Here's how the part is built. I have some questions about the finished solid (model axes, mm). A direction names the side the tool comes from. Give positions to 0.01 mm unless a question says otherwise; leave off trailing zeros. Order: outer loops, then holes, each group sorted by start corner. A loop starts at its lowest first (then second) coordinate and runs counter-clockwise, first axis right, second up. Notation, with made-up numbers: (88, 37) - (110, 37) arc R9 cw to (110, 43) - close; hole circle Ø4 at (11, 40). An arc over 180 degrees is marked (long way). One line per question, with ' | ' between items.
from build123d import *

# Parameters (mm, degrees)
SKETCH1_W                                 = 16
SKETCH1_H                                 = 16
BASE_DEPTH                                = 55
SKETCH2_W                                 = 2
SKETCH2_H                                 = 16
RODSLOT_DEPTH                             = 17
F_5_1_5_1_FREE_HOLE_FOR_SCREW_D           = 5.1
F_5_1_5_1_FREE_HOLE_FOR_SCREW_DEPTH       = 7.5
F_5_1_5_1_FREE_HOLE_FOR_SCREW_CSINK_D     = 6.1
F_5_1_5_1_FREE_HOLE_FOR_SCREW_CSINK_ANGLE = 90
F_5_1_5_1_FREE_HOLE_FOR_SCREW_TIP         = 1.056244584
M5X0_8_TAPPED_HOLE_FOR_ROD_SCREW_D        = 4.2
M5X0_8_TAPPED_HOLE_FOR_ROD_SCREW_DEPTH    = 7.6381927
M5X0_8_TAPPED_HOLE_FOR_ROD_SCREW_TIP      = 1.2618073
F_10_2_10_2_ROD_HOLE_D                    = 10.2
SKETCH13_W                                = 20
SKETCH13_H                                = 2
ROD2SLOT_DEPTH                            = 17
F_10_2_10_2_ROD2_HOLE_D                   = 10.2
F_5_1_5_1_DIAMETER_HOLE1_D                = 5.1
F_5_1_5_1_DIAMETER_HOLE1_DEPTH            = 7.5
F_5_1_5_1_DIAMETER_HOLE1_CSINK_D          = 6.1
F_5_1_5_1_DIAMETER_HOLE1_CSINK_ANGLE      = 90
F_5_1_5_1_DIAMETER_HOLE1_TIP              = 1.056244584
M5X0_8_TAPPED_HOLE1_D                     = 4.2
M5X0_8_TAPPED_HOLE1_DEPTH                 = 7.6381927
M5X0_8_TAPPED_HOLE1_TIP                   = 1.2618073


with BuildPart() as part:
    # Sketch1 → Base (new body)
    with BuildSketch(Plane.XY):
        Rectangle(SKETCH1_W, SKETCH1_H)
    extrude(amount=BASE_DEPTH)

    # Sketch2 → RodSlot (cut, through all)
    with BuildSketch(Plane(origin=(0, 8, 0), x_dir=(1, 0, 0), z_dir=(0, 1, 0))):
        with Locations((0, -47)):
            Rectangle(SKETCH2_W, SKETCH2_H)
    extrude(amount=-RODSLOT_DEPTH, mode=Mode.SUBTRACT)

    # Ø5.1 (5.1) free hole for screw
    with Locations(Plane(origin=(8, 0, 0), x_dir=(0, 0, -1), z_dir=(1, 0, 0))):
        with Locations((-50, 0)):
            CounterSinkHole(F_5_1_5_1_FREE_HOLE_FOR_SCREW_D / 2, F_5_1_5_1_FREE_HOLE_FOR_SCREW_CSINK_D / 2, depth=F_5_1_5_1_FREE_HOLE_FOR_SCREW_DEPTH, counter_sink_angle=F_5_1_5_1_FREE_HOLE_FOR_SCREW_CSINK_ANGLE)
            with Locations((0, 0, -(F_5_1_5_1_FREE_HOLE_FOR_SCREW_DEPTH + F_5_1_5_1_FREE_HOLE_FOR_SCREW_TIP / 2))):  # 135° drill point
                Cone(0, F_5_1_5_1_FREE_HOLE_FOR_SCREW_D / 2, F_5_1_5_1_FREE_HOLE_FOR_SCREW_TIP, mode=Mode.SUBTRACT)

    # M5x0.8 Tapped Hole for rod screw
    with Locations(Plane.ZY.offset(8)):
        with Locations((50, 0)):
            Hole(M5X0_8_TAPPED_HOLE_FOR_ROD_SCREW_D / 2, depth=M5X0_8_TAPPED_HOLE_FOR_ROD_SCREW_DEPTH)
            with Locations((0, 0, -(M5X0_8_TAPPED_HOLE_FOR_ROD_SCREW_DEPTH + M5X0_8_TAPPED_HOLE_FOR_ROD_SCREW_TIP / 2))):  # 118° drill point
                Cone(0, M5X0_8_TAPPED_HOLE_FOR_ROD_SCREW_D / 2, M5X0_8_TAPPED_HOLE_FOR_ROD_SCREW_TIP, mode=Mode.SUBTRACT)

    # Ø10.2 (10.2) Rod Hole (through all)
    with Locations(Plane(origin=(0, 8, 0), x_dir=(1, 0, 0), z_dir=(0, 1, 0))):
        with Locations((0, -35)):
            Hole(F_10_2_10_2_ROD_HOLE_D / 2)

    # Sketch13 → Rod2Slot (cut, through all)
    with BuildSketch(Plane.ZY.offset(8)):
        with Locations((10, 0)):
            Rectangle(SKETCH13_W, SKETCH13_H)
    extrude(amount=-ROD2SLOT_DEPTH, mode=Mode.SUBTRACT)

    # Ø10.2 (10.2) Rod2 Hole (through all)
    with Locations(Plane(origin=(-8, 0, 0), x_dir=(0, 1, 0), z_dir=(-1, 0, 0))):
        with Locations((0, -20)):
            Hole(F_10_2_10_2_ROD2_HOLE_D / 2)

    # Ø5.1 (5.1) Diameter Hole1
    with Locations(Plane(origin=(0, 8, 0), x_dir=(0, 0, -1), z_dir=(0, 1, 0))):
        with Locations((-5, 0)):
            CounterSinkHole(F_5_1_5_1_DIAMETER_HOLE1_D / 2, F_5_1_5_1_DIAMETER_HOLE1_CSINK_D / 2, depth=F_5_1_5_1_DIAMETER_HOLE1_DEPTH, counter_sink_angle=F_5_1_5_1_DIAMETER_HOLE1_CSINK_ANGLE)
            with Locations((0, 0, -(F_5_1_5_1_DIAMETER_HOLE1_DEPTH + F_5_1_5_1_DIAMETER_HOLE1_TIP / 2))):  # 135° drill point
                Cone(0, F_5_1_5_1_DIAMETER_HOLE1_D / 2, F_5_1_5_1_DIAMETER_HOLE1_TIP, mode=Mode.SUBTRACT)

    # M5x0.8 Tapped Hole1
    with Locations(Plane(origin=(0, -8, 0), x_dir=(-1, 0, 0), z_dir=(0, -1, 0))):
        with Locations((0, -5)):
            Hole(M5X0_8_TAPPED_HOLE1_D / 2, depth=M5X0_8_TAPPED_HOLE1_DEPTH)
            with Locations((0, 0, -(M5X0_8_TAPPED_HOLE1_DEPTH + M5X0_8_TAPPED_HOLE1_TIP / 2))):  # 118° drill point
                Cone(0, M5X0_8_TAPPED_HOLE1_D / 2, M5X0_8_TAPPED_HOLE1_TIP, mode=Mode.SUBTRACT)


solid = part.part
1) I want a section at D-D (z = 50). List the corners of the cut face in (x, y) for me.
Model answer:
outline: (-8, -8) - (-1, -8) - (-1, -2.1) - (-8, -2.1) - close; (-8, 2.1) - (-1, 2.1) - (-1, 8) - (-8, 8) - close; (1, -8) - (8, -8) - (8, -3.05) - (7.5, -2.55) - (1, -2.55) - close; (1, 2.55) - (7.5, 2.55) - (8, 3.05) - (8, 8) - (1, 8) - close
2) I want a section at B-B (z = 12.5). List the corners of the cut face in (x, y) for me, plus the area to 3 significant figures.
Model answer:
outline: (-8, -8) - (8, -8) - (8, -1) - (-8, -1) - close; (-8, 1) - (8, 1) - (8, 8) - (-8, 8) - close | area: 224 mm2
3) Thinking about a two-plate mould opening in Z: for faces 1 (the face through (1, 0, 46)), 2 (the face through (0, -4, 0)), 3 (the face through (4, 0, 55)), 4 (the face through (-0.21, -0.112, 29.904)), which applies, +Z half, -Z half, draft (parallel to the pull), parting line (faces both ways), or undercut?
Model answer:
face 1: draft | face 2: -Z half | face 3: +Z half | face 4: undercut
4) I want a section at C-C (x = 0). List the corners of the cut face in (y, z) for me.
Model answer:
outline: (-8, 0) - (-1, 0) - (-1, 2.9) - (-8, 2.9) - close; (-8, 7.1) - (-1, 7.1) - (-1, 15) arc R5.1 cw (long way) to (1, 15) - (1, 7.55) - (7.5, 7.55) - (8, 8.05) - (8, 29.9) - (-8, 29.9) - close; (1, 0) - (8, 0) - (8, 1.95) - (7.5, 2.45) - (1, 2.45) - close
5) Please list where these lines run through material, in increasing order: L1, parallel to Z at x = 5.5, y = 0; L2, parallel to Z at x = 0, y = -4.5; L3, parallel to Z at x = 0, y = -4.
Model answer:
L1: z = 25.1 to 47.45, 52.55 to 55 | L2: z = 0 to 2.9, 7.1 to 17.6, 22.4 to 29.9 | L3: z = 0 to 2.9, 7.1 to 16.84, 23.16 to 29.9
6) On a 3-axis mill with a long thin cutter (end or side, diameter ignored), from which of +Z, -Z, +X, -X, +Y, -Y can I reach the whole of each face in a straight line? I mean faces 5 (the face through (-0.1, -1, 7.4)), 6 (the face through (-1, 0.1, 47.6)), 7 (the face through (4.204, 0.112, 47.452)). Say none if no direction works.
Model answer:
face 5: -Z, +X, -X | face 6: +Z, +Y, -Y | face 7: +X
7) I want a section at A-A (y = -4.5). List the corners of the cut face in (x, z) for me, plus the area to 3 significant figures.
Model answer:
outline: (-8, 0) - (8, 0) - (8, 17.6) - (-8, 17.6) - close; (-8, 22.4) - (8, 22.4) - (8, 55) - (1, 55) - (1, 40) arc R5.1 cw (long way) to (-1, 40) - (-1, 55) - (-8, 55) - close; hole circle Ø4.2 at (0, 5) | area: 678 mm2
8) I'm going to push flat-ended pins straight in: P1, Ø4.5, axis at x = 0.5, z = 7.5, coming from the +Y side; P2, Ø5, axis at y = 0, z = 50, coming from the +X side. Where does each tip first touch, or does it pass through?
Model answer:
P1: stops at y = 8 | P2: stops at x = -1
